Build history of the part. All positions in model axes, mm. Face numbers are marked on the shaded views. A direction names the side the tool comes from. Round coordinates to 2 decimals unless told otherwise and drop trailing zeros. Loops run counter-clockwise (first coordinate to the right, second up) from the corner with the lowest first, then second, coordinate; pieces in that order, holes last. Notation, with made-up numbers: (-7.5, 71) -> (1.5, 71) arc R23 ccw to (1.5, 81) -> close; hole circle Ø9 at (-14, -11). An arc over 180 degrees is marked (long way). Put each result on its own line as item: value. Start each with the question number.
```python
from build123d import *

# Parameters (mm, degrees)
F0_W     = 28.575
F0_H     = 12.7
F0_W_2   = 12.7
F0_H_2   = 38.1
F1_DEPTH = 25.4
F2_W     = 12.7
F2_H     = 12.7
F4_W     = 12.7
F4_H     = 12.7
F7_DEPTH = 25.4
F9_DEPTH = 25.4


with BuildPart() as f1:
    # F0 (on Top) → F1 (new body)
    with BuildSketch(Plane.XY):
        with Locations((-36.5125, -44.45)):
            Rectangle(F0_W, F0_H)
        with Locations((-15.875, -19.05)):
            Rectangle(F0_W_2, F0_H_2)
        with BuildLine():
            ThreePointArc((22.225, 0), (0, 22.225), (-22.225, 0))
            Line((-22.225, 0), (-9.525, 0))
            ThreePointArc((-9.525, 0), (0, 9.525), (9.525, 0))
            Line((9.525, 0), (22.225, 0))
        make_face()
        with Locations((15.875, -6.35)):
            Rectangle(F0_W_2, F0_H)
        with Locations((15.875, -19.05)):
            Rectangle(F0_W_2, F0_H)
        with Locations((36.5125, -19.05)):
            Rectangle(F0_W, F0_H)
        with Locations((-15.875, -44.45)):
            Rectangle(F0_W_2, F0_H)
    extrude(amount=F1_DEPTH)

    # F2 (on face) → F3 (revolve)
    with BuildSketch(Plane(origin=(-50.8, 0, 0), x_dir=(0, -1, 0), z_dir=(-1, 0, 0))):
        with Locations((44.45, 19.05)):
            Rectangle(F2_W, F2_H)
    revolve(axis=Axis((-50.8, -44.45, 12.7), (0, -1, 0)))

    # F4 (on face) → F5 (revolve)
    with BuildSketch(Plane.YZ.offset(50.8)):
        with Locations((-19.05, 19.05)):
            Rectangle(F4_W, F4_H)
    revolve(axis=Axis((50.8, -19.05, 12.7), (0, 1, 0)))

    # F6 (on face) → F7 (cut)
    with BuildSketch(Plane.XZ.offset(25.4)):
        with BuildLine():
            ThreePointArc((57.15, 12.7), (55.290128, 17.190128), (50.8, 19.05))
            Line((50.8, 19.05), (50.8, 6.35))
            ThreePointArc((50.8, 6.35), (55.290128, 8.209872), (57.15, 12.7))
        make_face()
        with BuildLine():
            Line((50.8, 6.35), (50.8, 19.05))
            ThreePointArc((50.8, 19.05), (44.45, 12.7), (50.8, 6.35))
        make_face()
    extrude(amount=-F7_DEPTH, mode=Mode.SUBTRACT)

    # F8 (on face) → F9 (cut)
    with BuildSketch(Plane.XZ.offset(50.8)):
        with BuildLine():
            ThreePointArc((-44.45, 12.7), (-46.309872, 17.190128), (-50.8, 19.05))
            Line((-50.8, 19.05), (-50.8, 6.35))
            ThreePointArc((-50.8, 6.35), (-46.309872, 8.209872), (-44.45, 12.7))
        make_face()
        with BuildLine():
            Line((-50.8, 6.35), (-50.8, 19.05))
            ThreePointArc((-50.8, 19.05), (-57.15, 12.7), (-50.8, 6.35))
        make_face()
    extrude(amount=-F9_DEPTH, mode=Mode.SUBTRACT)


solid = f1.part
```
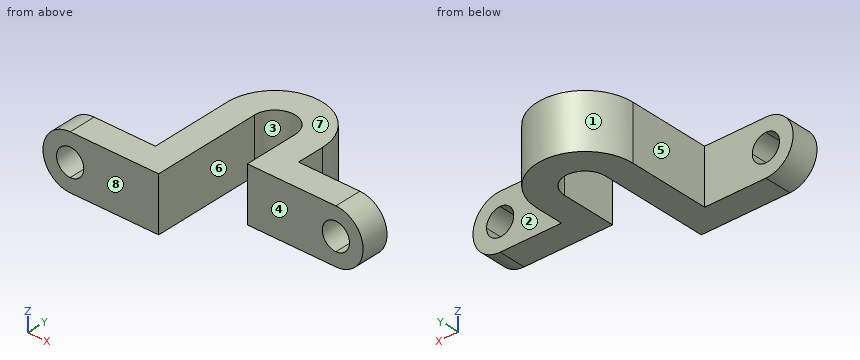
Item 1: Pull direction X, two halves, no side cores. Call the marked faces 1, 2 and 3: +X half, -X half, draft (parallel to the pull), parting line (faces both ways), or undercut.
Item 2: Cut at A-A on y = -23. Write the cut outline in (x, z) (3 decimals).
Item 3: Cut at C-C on y = -44.5. Write the cut outline in (x, z) (3 decimals), then the cut area to 3 significant figures.
Item 4: Wall check: line 1 (X direction, y = -16.5, z = 14.5) (3 decimals); line 2 (X direction, y = -12, z = 18.75) (3 decimals); line 3 (X direction, y = -35.5, z = 4.75) (3 decimals). Give the ranges that are in metal, low to high. Write a range as from..to.
Item 5: Drop flat-ended pins along their axis: pin 1 (4 mm diameter, centred on y = -3.5, z = 7.5, fed in from +X) (3 decimals); pin 2 (5 mm diameter, centred on y = -13.5, z = 19, fed in from +X); pin 3 (1.5 mm diameter, centred on x = 47, y = -14, fed in from -Z); pin 4 (7.5 mm diameter, centred on y = -20.5, z = 13.5, fed in from -X) (3 decimals). Give the stop position or say it passes through.
Item 6: Cut at D-D on z = 17.5. Write the cut outline in (x, y) (3 decimals), then the cut area to 3 significant figures.
Item 7: 3-axis set-ups, long thin cutter, end or side, ignore diameter. For the marked faces 4, 5, 6, 7 and 8: which of +Z, -Z, +X, -X, +Y, -Y reach the whole face in a straight line?
Item 8: Cut at B-B on y = -7.5. Write the cut outline in (x, z) (3 decimals), then the cut area to 3 significant figures.
Ans:
1. face 1: parting line
1. face 2: draft
1. face 3: undercut
2. outline: (-22.225, 0) -> (-9.525, 0) -> (-9.525, 25.4) -> (-22.225, 25.4) -> close; (9.525, 0) -> (50.8, 0) arc R12.7 ccw to (50.8, 25.4) -> (9.525, 25.4) -> close; hole circle Ø12.7 at (50.8, 12.7)
3. outline: (-50.8, 0) -> (-9.525, 0) -> (-9.525, 25.4) -> (-50.8, 25.4) arc R12.7 ccw to start; hole circle Ø12.7 at (-50.8, 12.7)
3. area: 1,180 mm2
4. line 1: x = -22.225..-9.525, 9.525..44.71, 56.89..63.372
4. line 2: x = -22.225..-9.525, 9.525..22.225
4. line 3: x = -22.225..-9.525
5. pin 1: stops at x = 22.225
5. pin 2: stops at x = 62.92
5. pin 3: stops at z = 0
5. pin 4: stops at x = -22.225
6. outline: (-62.558, -50.8) -> (-54.957, -50.8) -> (-54.957, -38.1) -> (-62.558, -38.1) -> close; (-46.643, -50.8) -> (-9.525, -50.8) -> (-9.525, 0) arc R9.525 cw to (9.525, 0) -> (9.525, -25.4) -> (46.643, -25.4) -> (46.643, -12.7) -> (22.225, -12.7) -> (22.225, 0) arc R22.225 ccw to (-22.225, 0) -> (-22.225, -38.1) -> (-46.643, -38.1) -> close; (54.957, -25.4) -> (62.558, -25.4) -> (62.558, -12.7) -> (54.957, -12.7) -> close
6. area: 2,410 mm2
7. face 4: +Z, -Z, +X, -Y
7. face 5: +Z, -Z, -X, +Y
7. face 6: +Z, -Z, -Y
7. face 7: +Z, +X, -X, +Y, -Y
7. face 8: +Z, -Z, +X, -X, -Y
8. outline: (-22.225, 0) -> (-9.525, 0) -> (-9.525, 25.4) -> (-22.225, 25.4) -> close; (9.525, 0) -> (22.225, 0) -> (22.225, 25.4) -> (9.525, 25.4) -> close
8. area: 645 mm2
